For this review, take the finished solid that the model builds, in its own axes (mm). A direction names the side the tool comes from. Give positions to 0.01 mm unless a question says otherwise; leave off trailing zeros. Write each loop counter-clockwise with the first axis right and the second up, starting at its lowest first coordinate (ties: lowest second). Pieces come first, ordered by that corner, then holes.
1) For P1, Ø4, axis at x = 0, y = 15, coming from the -Z side; P2, Ø1, axis at x = 3, z = -3, coming from the +Y side; P3, Ø6, axis at y = 8, z = 3.5, coming from the +X side; P4, Ø1, axis at x = 4.5, z = 3, coming from the -Y side, all flat-tipped, find the tip position at first contact; note any pin that passes through.
2) We need section D-D on y = 4. Give the boundary of the cut face in (x, z), and give its area (3 significant figures).
3) Machinability: for faces 1 (the face through (4.3, 12.9, 0)), 2 (the face through (0, 2, 3)), 3 (the face through (0, 13, -1.9)), 4 (the face through (-4.3, 12.9, 0)), which of the approach directions +Z, -Z, +X, -X, +Y, -Y give a long, thin tool a straight path to every point of the face, cutting with its end or side? Answer none if there is none.
4) Draft analysis for pull direction X (two halves, no side actions). For faces 5 (the face through (0.672, 16.054, 0.027)), 6 (the face through (0, 2, -3)), 7 (the face through (6.5, 6.6, -0.1)), state which applies: pulls with the +X half, pulls with the -X half, needs draft (parallel to the pull), parting line crosses it, or undercut.
5) We need section A-A on x = 0.75. Give the boundary of the cut face in (y, z), and give its area (3 significant figures).
6) We need section C-C on z = 0. Give the boundary of the cut face in (x, y), and give its area (3 significant figures).
7) We need section B-B on y = 15. Give the boundary of the cut face in (x, z).
8) Wall thickness on line 1 along Y through (x, z) = (0, 4.25); line 2 along Y through (x, z) = (0, -0.45); line 3 along Z through (x, y) = (3.5, 4): over which ranges is each line inside the solid? List them lowest first.
from build123d import *

# Parameters (mm, degrees)
EXTRUDE_1_DEPTH     = 8
EXTRUDE_2_DEPTH     = 10
SKETCH_3_R          = 1.25
CUT_EXTRUDE_1_DEPTH = 6
SKETCH_4_W          = 25.11911159
SKETCH_4_H          = 6
CUT_EXTRUDE_2_DEPTH = 6
SKETCH_5_R          = 1.25
CUT_EXTRUDE_3_DEPTH = 22.592822882


with BuildPart() as part:
    # 草图1 → 凸台-拉伸1 (new body)
    with BuildSketch(Plane(origin=(0, 0, 0), x_dir=(1, 0, 0), z_dir=(0, 1, 0))):
        with BuildLine():
            Line((-1.5, 5), (1.5, 5))
            ThreePointArc((1.5, 5), (6.5, 0), (1.5, -5))
            Line((1.5, -5), (-1.5, -5))
            ThreePointArc((-1.5, -5), (-6.5, 0), (-1.5, 5))
        make_face()
    extrude(amount=EXTRUDE_1_DEPTH)

    # 草图2 → 凸台-拉伸2 (add)
    with BuildSketch(Plane(origin=(0, 8, 0), x_dir=(1, 0, 0), z_dir=(0, 1, 0))):
        with BuildLine():
            Line((-2.4, 1.9), (2.4, 1.9))
            ThreePointArc((2.4, 1.9), (4.3, 0), (2.4, -1.9))
            Line((2.4, -1.9), (-2.4, -1.9))
            ThreePointArc((-2.4, -1.9), (-4.3, 0), (-2.4, 1.9))
        make_face()
    extrude(amount=EXTRUDE_2_DEPTH)

    # 草图3 → 切除-拉伸1 (cut)
    with BuildSketch(Plane.XY.offset(1.9)):
        with Locations((0, 15)):
            Circle(SKETCH_3_R)
    extrude(amount=-CUT_EXTRUDE_1_DEPTH, mode=Mode.SUBTRACT)

    # 草图4 → 切除-拉伸2 (cut)
    with BuildSketch(Plane.XZ):
        Rectangle(SKETCH_4_W, SKETCH_4_H)
    extrude(amount=-CUT_EXTRUDE_2_DEPTH, mode=Mode.SUBTRACT)

    # 草图5 → 切除-拉伸3 (cut, through all)
    with BuildSketch(Plane.XY.offset(5)):
        with Locations((0, 4)):
            Circle(SKETCH_5_R)
    extrude(amount=-CUT_EXTRUDE_3_DEPTH, mode=Mode.SUBTRACT)


solid = part.part
Results list:
1. P1: stops at z = -1.9
1. P2: stops at y = 8
1. P3: stops at x = 6.47
1. P4: stops at y = 0
2. outline: (-5.5, -3) arc R5 ccw to (-1.5, -5) - (-1.25, -5) - (-1.25, -3) - close; (-5.5, 3) - (-1.25, 3) - (-1.25, 5) - (-1.5, 5) arc R5 ccw to start; (1.25, -5) - (1.5, -5) arc R5 ccw to (5.5, -3) - (1.25, -3) - close; (1.25, 3) - (5.5, 3) arc R5 ccw to (1.5, 5) - (1.25, 5) - close
2. area: 24.4 mm2
3. face 1: +X, +Y
3. face 2: +X, -X, -Y
3. face 3: -Z, +X, -X, +Y
3. face 4: -X, +Y
4. face 5: undercut
4. face 6: needs draft
4. face 7: pulls with the +X half
5. outline: (0, -5) - (3, -5) - (3, -3) - (0, -3) - close; (0, 3) - (3, 3) - (3, 5) - (0, 5) - close; (5, -5) - (8, -5) - (8, -1.9) - (14, -1.9) - (14, 1.9) - (8, 1.9) - (8, 5) - (5, 5) - (5, 3) - (6, 3) - (6, -3) - (5, -3) - close; (16, -1.9) - (18, -1.9) - (18, 1.9) - (16, 1.9) - close
5. area: 66.4 mm2
6. outline: (-6.5, 6) - (6.5, 6) - (6.5, 8) - (4.3, 8) - (4.3, 18) - (-4.3, 18) - (-4.3, 8) - (-6.5, 8) - close; hole circle Ø2.5 at (0, 15)
6. area: 107 mm2
7. outline: (-2.4, -1.9) - (-1.25, -1.9) - (-1.25, 1.9) - (-2.4, 1.9) arc R1.9 ccw to start; (1.25, -1.9) - (2.4, -1.9) arc R1.9 ccw to (2.4, 1.9) - (1.25, 1.9) - close
8. line 1: y = 0 to 2.75, 5.25 to 8
8. line 2: y = 6 to 13.75, 16.25 to 18
8. line 3: z = -4.58 to -3, 3 to 4.58
